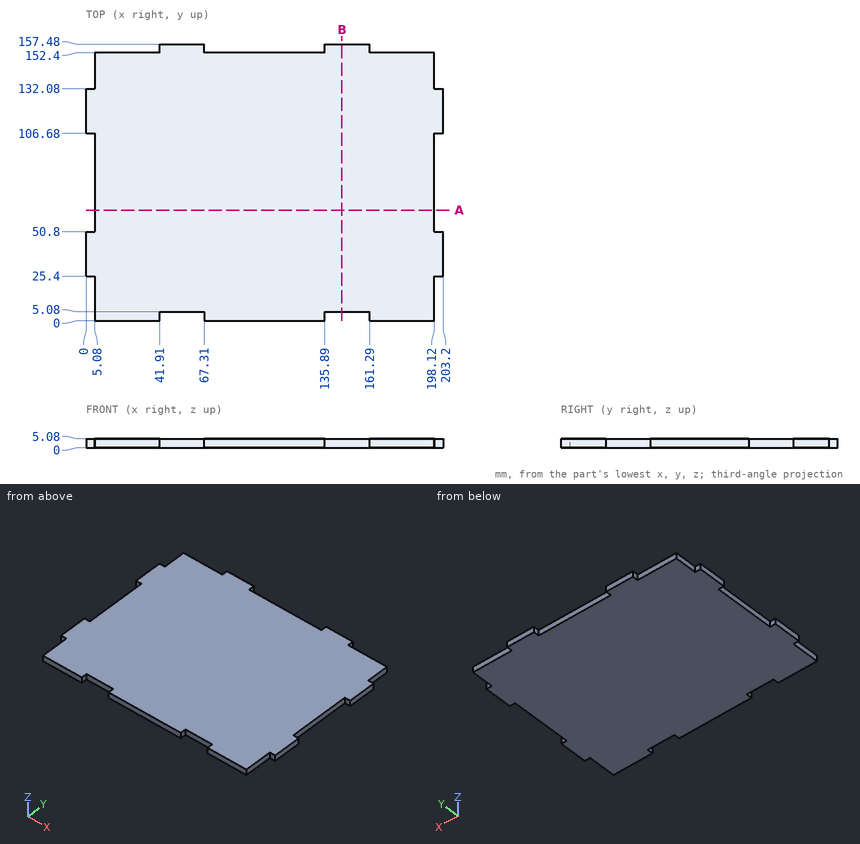
Answer from the drawing. Dimensions are ordinates in mm from the lowest x, y and z of the part. Coordinates: 2 decimals unless noted, no trailing zeros. Write each loop counter-clockwise with the first axis right and the second up, starting at its lowest first coordinate (ties: lowest second). Pieces come first, ordered by that corner, then holes. Notation, with made-up numbers: M -20.5,59.25 L 0.5,59.25 A27 cw 0.5,87.25 Z; hole C 11.25,4 d11. An arc over 180 degrees is marked long. Use a Markdown table: item, result.
Q1. The part is cut by section B-B, the plane x = 145.5. Write down the section's boundary in (y, z).
Answer block:
| item | result |
|---|---|
| outline | M 5.08,0 L 157.48,0 L 157.48,5.08 L 5.08,5.08 Z |
Q2. The part is cut by section A-A, the plane y = 63. Write down the section's boundary in (x, z), then the cut area to 3 significant figures.
Answer block:
| item | result |
|---|---|
| outline | M 5.08,0 L 198.12,0 L 198.12,5.08 L 5.08,5.08 Z |
| area | 981 mm2 |
Q3. Each of these flat-tipped pins is pushed along its axis until it touches: pin 1 Ø1.5 at (x, z) = (150.5, 3.5) entering from -Y; pin 2 Ø2.5 at (y, z) = (4, 1.5) entering from +X; pin 3 Ø2.5 at (x, z) = (179.5, 1.5) entering from +Y. Where does it stop, or does it pass through?
Answer block:
| item | result |
|---|---|
| pin 1 | stops at y = 5.08 |
| pin 2 | stops at x = 198.12 |
| pin 3 | stops at y = 152.4 |
Q4. Straight lines are drawn through the part: L1, parallel to X at y = 19, z = 2.9; L2, parallel to Y at x = 112, z = 1.9; L3, parallel to Y at x = 158, z = 1.95. For each, find the intervals that lie inside material, in ascending order. Write a range as [from, to].
Answer block:
| item | result |
|---|---|
| L1 | x = [5.08, 198.12] |
| L2 | y = [0, 152.4] |
| L3 | y = [5.08, 157.48] |
